Check sheet for the drawn part. Datum: minimum x, y, z corner. Units: mm. A direction names the side the tool comes from. Give positions to 0.01 mm unless a question says otherwise; leave off trailing zeros. Order: outer loops, then holes, each group sorted by start corner. A loop starts at its lowest first (then second) coordinate and runs counter-clockwise, first axis right, second up. Notation, with made-up numbers: (40.25, 89.25) -> (76.25, 89.25) arc R30 cw to (76.25, 112.25) -> close; hole circle Ø4 at (-6.5, 25). An arc over 180 degrees is marked (long way). One line per question, with ' | ' between items. Start each with the question number.
Q1. Section check C-C on z = 18. Record the cut outline in (x, y).
Q2. Section check D-D on z = 25. Record the cut outline in (x, y), plus the area to 3 significant figures.
Q3. Mould release check, pull along Z, two halves, no side actions. Record for the marked faces 1, 2 and 3: released by +Z, released by -Z, zero draft, split by the parting line, or undercut.
Q4. Section check A-A on x = 27. Record the cut outline in (y, z).
Q5. Go/stop test with a flat-tipped pin: pin 1 (1.5 mm diameter, centred on y = 1.5, z = 18.5, fed in from -X). Record where the tip stops, or that it passes through.
Q6. Material ranges on probe 1 along X at (y, z) = (0.95, 22); probe 2 along Z at (x, y) = (27, 2.7); probe 3 along X at (y, z) = (4.2, 24.75), recorded low to high. Write a range as [from, to].
Q7. Section check B-B on y = 1.8. Record the cut outline in (x, z), plus the area to 3 significant figures.
Q8. Access from +Z, -Z, +X, -X, +Y, -Y to the whole of each face (thin tool, end or side, straight path). Record for the marked faces 4, 5 and 6.
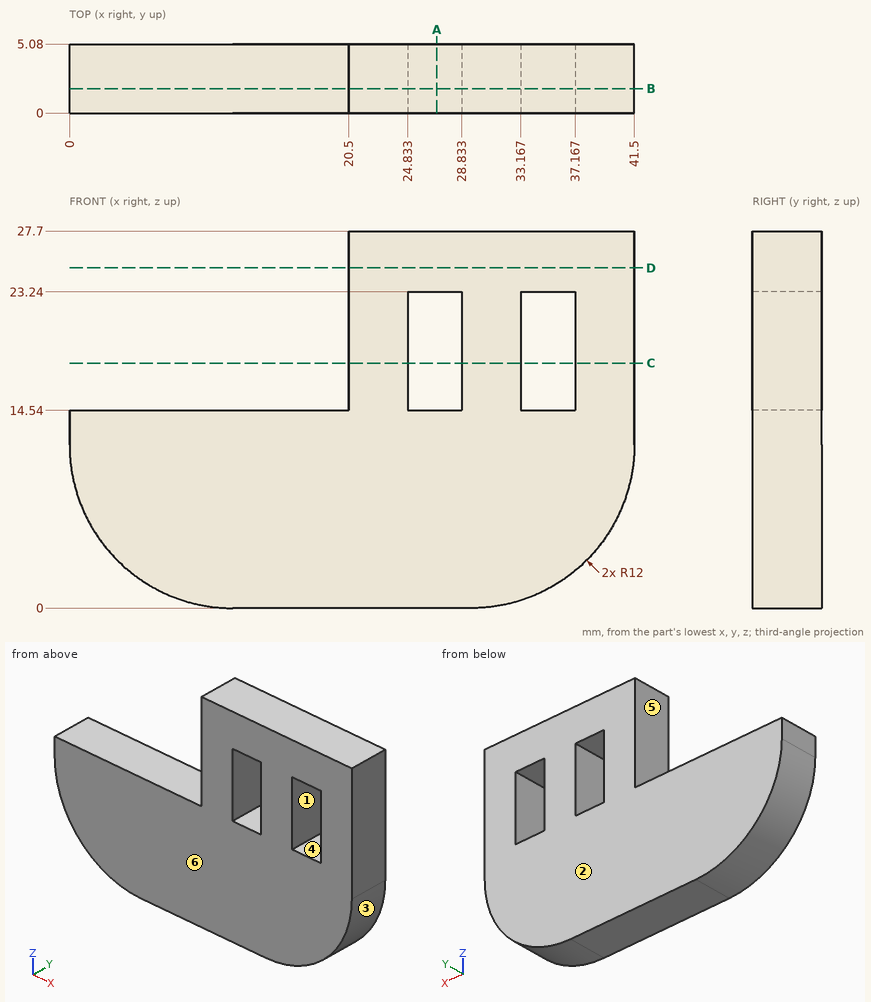
Filled in:
1) outline: (20.5, 0) -> (24.83, 0) -> (24.83, 5.08) -> (20.5, 5.08) -> close; (28.83, 0) -> (33.17, 0) -> (33.17, 5.08) -> (28.83, 5.08) -> close; (37.17, 0) -> (41.5, 0) -> (41.5, 5.08) -> (37.17, 5.08) -> close
2) outline: (20.5, 0) -> (41.5, 0) -> (41.5, 5.08) -> (20.5, 5.08) -> close | area: 107 mm²
3) face 1: undercut | face 2: zero draft | face 3: released by -Z
4) outline: (0, 0) -> (5.08, 0) -> (5.08, 14.54) -> (0, 14.54) -> close; (0, 23.24) -> (5.08, 23.24) -> (5.08, 27.7) -> (0, 27.7) -> close
5) pin 1: x = 20.5
6) probe 1: [20.5, 24.83], [28.83, 33.17], [37.17, 41.5] | probe 2: [0, 14.54], [23.24, 27.7] | probe 3: [20.5, 41.5]
7) outline: (0, 12) arc R12 ccw to (12, 0) -> (29.5, 0) arc R12 ccw to (41.5, 12) -> (41.5, 27.7) -> (20.5, 27.7) -> (20.5, 14.54) -> (0, 14.54) -> close; hole (24.83, 14.54) -> (28.83, 14.54) -> (28.83, 23.24) -> (24.83, 23.24) -> close; hole (33.17, 14.54) -> (37.17, 14.54) -> (37.17, 23.24) -> (33.17, 23.24) -> close | area: 748 mm²
8) face 4: +Y, -Y | face 5: +Z, -X, +Y, -Y | face 6: +Z, -Z, +X, -X, -Y
